Part model, mm, in its own coordinate system. Round coordinates to 2 decimals unless told otherwise and drop trailing zeros. Loops run counter-clockwise (first coordinate to the right, second up) from the corner with the lowest first, then second, coordinate; pieces in that order, holes last.
from build123d import *

# Parameters (mm, degrees)
SKETCH1_R           = 3.3235
BOSS_EXTRUDE1_DEPTH = 7.7
CHAMFER1_SIZE       = 0.5


with BuildPart() as part:
    # Sketch1 → Boss-Extrude1 (new body)
    with BuildSketch(Plane.XY):
        Polygon((3.695041723, 6.4), (-3.695041723, 6.4), (-7.390083446, 0), (-3.695041723, -6.4), (3.695041723, -6.4), (7.390083446, 0), align=None)
        Circle(SKETCH1_R, mode=Mode.SUBTRACT)
    extrude(amount=-BOSS_EXTRUDE1_DEPTH)

    # Sketch2 → Cut-Revolve1 (revolve, cut)
    with BuildSketch(Plane(origin=(0, 0, 0), x_dir=(1, 0, 0), z_dir=(0, 1, 0))):
        with BuildLine():
            Line((-7.390083446, 7.7), (-7.390083446, 4.3))
            ThreePointArc((-7.390083446, 4.3), (-7.05400145, 6.120027472), (-6.090083446, 7.7))
            Line((-6.090083446, 7.7), (-7.390083446, 7.7))
        make_face()
        with BuildLine():
            Line((-7.390083446, 0), (-7.390083446, 0.4))
            ThreePointArc((-7.390083446, 0.4), (-6.933916011, 0.103778026), (-6.4, 0))
            Line((-6.4, 0), (-7.390083446, 0))
        make_face()
    revolve(axis=Axis((0, 0, -8.105120256), (0, 0, 1)), mode=Mode.SUBTRACT)

    # Chamfer1
    chamfer1_edges = [part.edges().sort_by_distance(p)[0] for p in [
        (-3.3235, 0, -7.7),
        (-3.3235, 0, 0),
    ]]
    chamfer(chamfer1_edges, length=CHAMFER1_SIZE)


solid = part.part
1) Wall check: line 1 along Y through (x, z) = (0, -5.5); line 2 along Y through (x, z) = (-0.75, -6.25); line 3 along X through (y, z) = (-1.75, -4.75). Give the ranges that are in metal, low to high.
Values:
line 1: y = -6.4 to -3.32, 3.32 to 6.4
line 2: y = -6.4 to -3.24, 3.24 to 6.4
line 3: x = -6.38 to -2.83, 2.83 to 6.38
2) Mould opens along X. For faces 1 (the face through (3.07, -1.27, -3.8)), 2 (the face through (0, -6.4, -4)), 3 (the face through (-5.568, -3.155, -3.608)), 4 (the face through (5.52, -3.24, -3.61)) say: released by +X, released by -X, zero draft, split by the parting line, or undercut.
Values:
face 1: undercut
face 2: zero draft
face 3: released by -X
face 4: released by +X
3) Slice it at A-A, the plane z = -4. Give the cut face in (x, y), then the cut area to 3 significant figures.
Values:
outline: (-7.39, 0) - (-3.7, -6.4) - (3.7, -6.4) - (7.39, 0) - (3.7, 6.4) - (-3.7, 6.4) - close; hole circle Ø6.65 at (0, 0)
area: 107 mm2
4) Drop flat-ended pins along their axis: pin 1 Ø1.5 at (x, y) = (3.5, 2.5) entering from +Z; pin 2 Ø1.5 at (y, z) = (4.5, -3.5) entering from -X (3 decimals). Give the stop position or say it passes through.
Values:
pin 1: stops at z = 0
pin 2: stops at x = -5.225
